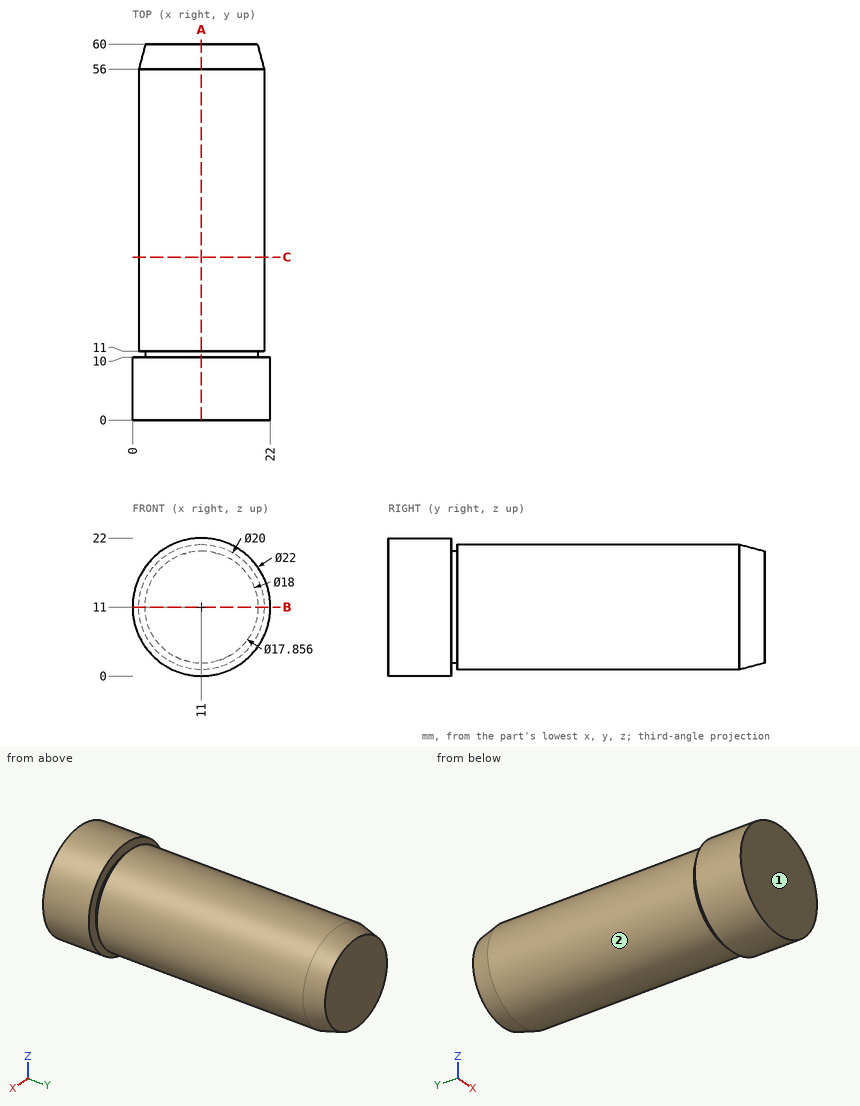
Input: dimensioned drawing with shaded views. Units: mm. Origin: part minimum x, y, z. A direction names the side the tool comes from. Coordinates: 2 decimals unless noted, no trailing zeros. Loops run counter-clockwise (first coordinate to the right, second up) from the corner with the lowest first, then second, coordinate; pieces in that order, holes last.
Q1. Section A-A, the plane x = 11. Return the cut outline in (y, z).
Results are:
outline: (0, 0) - (10, 0) - (10, 2) - (11, 2) - (11, 1) - (56, 1) - (60, 2.07) - (60, 19.93) - (56, 21) - (11, 21) - (11, 20) - (10, 20) - (10, 22) - (0, 22) - close
Q2. Section C-C, the plane y = 26. Return the cut outline in (x, z), and give its area (3 significant figures).
Results are:
outline: circle Ø20 at (11, 11)
area: 314 mm2
Q3. Section B-B, the plane z = 11. Return the cut outline in (x, y).
Results are:
outline: (0, 0) - (22, 0) - (22, 10) - (20, 10) - (20, 11) - (21, 11) - (21, 56) - (19.93, 60) - (2.07, 60) - (1, 56) - (1, 11) - (2, 11) - (2, 10) - (0, 10) - close
Q4. Line query: line 1 along X through (y, z) = (23.5, 11.25); line 2 along Z through (x, y) = (10.5, 21.5); line 3 along X through (y, z) = (28, 15.5). Output: solid intervals per line, ascending.
Results are:
line 1: x = 1 to 21
line 2: z = 1.01 to 20.99
line 3: x = 2.07 to 19.93
Q5. Contact query for flat-ended pins moving along their axis: pin 1 (4 mm diameter, centred on x = 18, y = 22.5, fed in from +Z); pin 2 (1.5 mm diameter, centred on x = 4.5, y = 26.5, fed in from -Z); pin 3 (8 mm diameter, centred on y = 35.5, z = 3, fed in from +X) (1 decimal). Output: stop coordinate, or through.
Results are:
pin 1: stops at z = 19.66
pin 2: stops at z = 2.82
pin 3: stops at x = 20.2
Q6. Set-up query: the marked faces 1 and 2. Return all of +Z, -Z, +X, -X, +Y, -Y with unobstructed straight access to the full face (end or side cutting, diameter ignored); none if empty.
Results are:
face 1: +Z, -Z, +X, -X, -Y
face 2: +Y
